Model file for the job. Use its own axes, mm. A direction names the side the tool comes from. Round coordinates to 2 decimals unless told otherwise and drop trailing zeros. Order: outer loops, then holes, each group sorted by start corner. A loop starts at its lowest first (then second) coordinate and runs counter-clockwise, first axis right, second up. Notation, with made-up numbers: M -29,-18 L -11,-18 A15 cw -11,-9 Z; hole C 31,22 d2. An arc over 180 degrees is marked long. Return JSON: item names as keys, results as strings. Group by question number.
Item 1: Pin check, flat tips, straight feed: pin 1 Ø5 at (x, y) = (-1, -10) entering from -Z; pin 2 Ø2 at (x, z) = (6.5, 92) entering from -Y (3 decimals); pin 3 Ø4 at (x, z) = (-13.5, 61) entering from +Y. Stop position of each tip, or through.
Item 2: Which spindle directions (+Z, -Z, +X, -X, +Y, -Y) get a long thin tool onto all of the face, cutting with end or side? Do faces 1 (the face through (1.42, -3.92, -4.85)), 2 (the face through (-3, 16, 3)), 3 (the face through (4, 5, 110)). Say none if no direction does.
Item 3: Probe line 1 along Z through (x, y) = (-14.5, -13); line 2 along Z through (x, y) = (-1, 6.5); line 3 along Z through (x, y) = (17.5, -9). List the from-to ranges inside material, lowest first.
Item 4: Slice it at A-A on z = 28. Write the cut outline in (x, y), then the cut area to 3 significant figures.
from build123d import *

# Parameters (mm, degrees)
SKETCH1_R           = 20
BOSS_EXTRUDE1_DEPTH = 3
CHAMFER1_SIZE       = 0.5
SKETCH2_R           = 16
BOSS_EXTRUDE2_DEPTH = 104
SKETCH3_R           = 20
BOSS_EXTRUDE3_DEPTH = 3
CHAMFER2_SIZE       = 0.5
SKETCH4_R           = 6
BOSS_EXTRUDE4_DEPTH = 4.85
SKETCH5_R           = 4
BOSS_EXTRUDE5_DEPTH = 8


with BuildPart() as part:
    # Sketch1 → Boss-Extrude1 (new body)
    with BuildSketch(Plane.XY):
        Circle(SKETCH1_R)
    extrude(amount=BOSS_EXTRUDE1_DEPTH)

    # Chamfer1
    chamfer1_edges = [part.edges().sort_by_distance(p)[0] for p in [
        (-20, 0, 0),
        (-20, 0, 3),
    ]]
    chamfer(chamfer1_edges, length=CHAMFER1_SIZE)

    # Sketch2 → Boss-Extrude2 (add)
    with BuildSketch(Plane.XY.offset(3)):
        with Locations(Location((0, 0, 0), (0, 0, 180))):
            Circle(SKETCH2_R)
    extrude(amount=BOSS_EXTRUDE2_DEPTH)

    # Sketch3 → Boss-Extrude3 (add)
    with BuildSketch(Plane.XY.offset(107)):
        Circle(SKETCH3_R)
    extrude(amount=BOSS_EXTRUDE3_DEPTH)

    # Chamfer2
    chamfer2_edges = [part.edges().sort_by_distance(p)[0] for p in [
        (-20, 0, 107),
        (-20, 0, 110),
    ]]
    chamfer(chamfer2_edges, length=CHAMFER2_SIZE)

    # Sketch4 → Boss-Extrude4 (add)
    with BuildSketch(Plane(origin=(0, 0, 0), x_dir=(-1, 0, 0), z_dir=(0, 0, -1))):
        Circle(SKETCH4_R)
    boss_extrude4 = extrude(amount=BOSS_EXTRUDE4_DEPTH)

    # Sketch5 → Boss-Extrude5 (add)
    with BuildSketch(Plane(origin=(0, 0, -4.85), x_dir=(-1, 0, 0), z_dir=(0, 0, -1))):
        Circle(SKETCH5_R)
    boss_extrude5 = extrude(amount=BOSS_EXTRUDE5_DEPTH)

    # Mirror2: Boss-Extrude4, Boss-Extrude5 across plane
    add(boss_extrude4.mirror(Plane(origin=(0, 0, 55), x_dir=(1, 0, 0), z_dir=(0, 0, -1))))
    add(boss_extrude5.mirror(Plane(origin=(0, 0, 55), x_dir=(1, 0, 0), z_dir=(0, 0, -1))))


solid = part.part
Output values:
{
 "1": {"pin 1": "z = 0", "pin 2": "y = -15.025", "pin 3": "y = 11.12"},
 "2": {"face 1": "-Z", "face 2": "none", "face 3": "+Z"},
 "3": {"line 1": "0 to 3, 107 to 110", "line 2": "0 to 110", "line 3": "0.18 to 2.82, 107.18 to 109.82"},
 "4": {"outline": "C 0,0 d32", "area": "804 mm²"}
}
